CAD build for the part. Positions are in the model's coordinates, mm. Round coordinates to 2 decimals unless told otherwise and drop trailing zeros. Order: outer loops, then holes, each group sorted by start corner. A loop starts at its lowest first (then second) coordinate and runs counter-clockwise, first axis right, second up. Notation, with made-up numbers: M 24.5,-27.75 L 74.5,-27.75 A22 cw 74.5,0.25 Z; hole C 34.5,73.25 d1. An arc over 180 degrees is marked long. Answer as CSV lines item,"result". Start each with the question number.
```python
from build123d import *

# Parameters (mm, degrees)
BOSS_EXTRUDE1_DEPTH = 2.5
SKETCH2_R           = 1.625
CUT_EXTRUDE1_DEPTH  = 2.5


with BuildPart() as part:
    # Sketch1 → Boss-Extrude1 (new body)
    with BuildSketch(Plane(origin=(0, 0, 0), x_dir=(1, 0, 0), z_dir=(0, 1, 0))):
        with BuildLine():
            Line((0, 4), (29, 4))
            ThreePointArc((29, 4), (33, 0), (29, -4))
            Line((29, -4), (0, -4))
            ThreePointArc((0, -4), (-4, 0), (0, 4))
        make_face()
    extrude(amount=BOSS_EXTRUDE1_DEPTH)

    # Sketch2 → Cut-Extrude1 (cut)
    with BuildSketch(Plane(origin=(0, 2.5, 0), x_dir=(1, 0, 0), z_dir=(0, 1, 0))):
        Circle(SKETCH2_R)
        with Locations((29, 0)):
            Circle(SKETCH2_R)
    extrude(amount=-CUT_EXTRUDE1_DEPTH, mode=Mode.SUBTRACT)


solid = part.part
```
Q1. Band-saw the part on A-A, the plane y = 2.1. Write the cut outline in (x, z) (3 decimals).
Q2. Mould opens along Z. For faces 1 (the flat face through (15, 1, 4)), 2 (the cylindrical face through (27.377, 1.268, -0.071)), 3 (the flat face through (15, 2.5, 0)) say: +Z half, -Z half, draft (parallel to the pull), parting line (faces both ways), or undercut.
Q3. Probe line 1 along X through (y, z) = (1.35, 0) (3 decimals); line 2 along Z through (x, y) = (0, 1.9) (3 decimals); line 3 along X through (y, z) = (1.1, 1). List the from-to ranges inside material, lowest first. Write a range as from..to.
Q4. Band-saw the part on D-D, the plane z = -2.75. Write the cut outline in (x, y).
Q5. Drop flat-ended pins along their axis: P1, Ø1.5, axis at y = 2, z = -3, coming from the -X side; P2, Ø1.5, axis at x = 19.5, z = -0.5, coming from the -Y side. Give the stop position or say it passes through.
Q6. Band-saw the part on C-C, the plane z = 2.5. Write the cut outline in (x, y), then the cut area to 3 significant figures.
Q7. Band-saw the part on B-B, the plane z = 0.5. Write the cut outline in (x, y), then the cut area to 3 significant figures.
Answer:
1,outline,"M 0,-4 L 29,-4 A4 ccw 29,4 L 0,4 A4 ccw Z; hole C 0,0 d3.25; hole C 29,0 d3.25"
2,face 1,"+Z half"
2,face 2,"undercut"
2,face 3,"draft"
3,line 1,"x = -4..-1.625, 1.625..27.375, 30.625..33"
3,line 2,"z = -4..-1.625, 1.625..4"
3,line 3,"x = -3.87..-1.28, 1.28..27.72, 30.28..32.87"
4,outline,"M -2.9,0 L 31.9,0 L 31.9,2.5 L -2.9,2.5 Z"
5,P1,"stops at x = -3.31"
5,P2,"stops at y = 0"
6,outline,"M -3.12,0 L 32.12,0 L 32.12,2.5 L -3.12,2.5 Z"
6,area,"88.1 mm^2"
7,outline,"M -3.97,0 L -1.55,0 L -1.55,2.5 L -3.97,2.5 Z; M 1.55,0 L 27.45,0 L 27.45,2.5 L 1.55,2.5 Z; M 30.55,0 L 32.97,0 L 32.97,2.5 L 30.55,2.5 Z"
7,area,"76.9 mm^2"
